Design review of the part built by this model. Coordinates are the model's own, in mm. A direction names the side the tool comes from. Coordinates: 2 decimals unless noted, no trailing zeros. Loops run counter-clockwise (first coordinate to the right, second up) from the corner with the lowest first, then second, coordinate; pieces in that order, holes last. Notation, with made-up numbers: (-1, 6) -> (50, 6) arc R37 ccw to (50, 43) -> close; hole circle Ø10 at (-35, -28.75). An arc over 180 degrees is marked (long way). One line per item, written item: value. Start each with the question number.
1. For probe 1 along Y at (x, z) = (0, 9.5); probe 2 along X at (y, z) = (-5.75, 33); probe 3 along Y at (x, z) = (3.25, 33.5), list the stretches that pass through material, from the lowest coordinate up.
2. Add section D-D on y = -5.5. Write out the cut boundary in (x, z), plus the area to 3 significant figures.
3. Machinability: for faces 1 (the cylindrical face through (0.07, 8.45, 18.54)), 2 (the flat face through (4.733, -4, 19)), 3 (the flat face through (-4.733, 4, 19)), 4 (the flat face through (-4.733, -4, 19)), 5 (the flat face through (4.733, 4, 19)), which of the approach directions +Z, -Z, +X, -X, +Y, -Y give a long, thin tool a straight path to every point of the face, cutting with its end or side? Answer none if there is none.
4. Draft analysis for pull direction X (two halves, no side actions). For faces 6 (the cylindrical face through (-5.458, -0.016, 19.063)), 7 (the cylindrical face through (-0.07, -8.45, 18.54)), 8 (the cylindrical face through (5.458, -0.016, 19.063)), 9 (the cylindrical face through (3.434, 1.081, 18.537)), state which applies: pulls with the +X half, pulls with the -X half, needs draft (parallel to the pull), parting line crosses it, or undercut.
5. Add section A-A on y = 0. Write out the cut boundary in (x, z), plus the area to 3 significant figures.
6. Insertion check: pin 1 (5 mm diameter, centred on y = 3, z = 11.5, fed in from +X); pin 2 (3 mm diameter, centred on y = -3, z = 21.5, fed in from -X); pin 3 (5 mm diameter, centred on y = 3, z = 13, fed in from -X); pin 4 (6 mm diameter, centred on x = 0, y = 0, fed in from +Z). Each pin has a flat end and moves straight along its axis. Give the tip position at first contact, or say it passes through.
7. Add section B-B on x = 0. Write out the cut boundary in (y, z).
8. Add section C-C on z = 26. Write out the cut boundary in (x, y) (3 decimals).
```python
from build123d import *

# Parameters (mm, degrees)
F0_R     = 3.6
F1_DEPTH = 37.6
F2_R     = 0.725
F3_DEPTH = 37.6


# Not quite as in the source:
# - a pattern or mirror of a feature is missing from the dataset's text; its kind, count and spacing are read off the source's solid


with BuildPart() as f1:
    # F0 (on Top) → F1 (new body)
    with BuildSketch(Plane.XY):
        with BuildLine():
            Line((4.7331279298, -7), (4.7331279298, 7))
            ThreePointArc((4.7331279298, 7), (0, 8.45), (-4.7331279298, 7))
            Line((-4.7331279298, 7), (-4.7331279298, -7))
            ThreePointArc((-4.7331279298, -7), (0, -8.45), (4.7331279298, -7))
        make_face()
        Circle(F0_R, mode=Mode.SUBTRACT)
    extrude(amount=F1_DEPTH)

    # F2 (on face) → F3 (join)
    with BuildSketch(Plane.XY.offset(37.6)):
        with Locations((4.7331279298, 0)):
            Circle(F2_R)
    f3 = extrude(amount=-F3_DEPTH)

    # F3_copies: F3 across plane
    add(f3.mirror(Plane(origin=(0, 0, 0), x_dir=(0, 0, -1), z_dir=(-1, 0, 0))))


solid = f1.part
```
Worked answers:
1. probe 1: y = -8.45 to -3.6, 3.6 to 8.45
1. probe 2: x = -4.73 to 4.73
1. probe 3: y = -7.8 to -1.55, 1.55 to 7.8
2. outline: (-4.73, 0) -> (4.73, 0) -> (4.73, 37.6) -> (-4.73, 37.6) -> close
2. area: 356 mm²
3. face 1: +Z, -Z, +Y
3. face 2: +Z, -Z, +X, -Y
3. face 3: +Z, -Z, -X, +Y
3. face 4: +Z, -Z, -X, -Y
3. face 5: +Z, -Z, +X, +Y
4. face 6: pulls with the -X half
4. face 7: parting line crosses it
4. face 8: pulls with the +X half
4. face 9: undercut
5. outline: (-5.46, 0) -> (-3.6, 0) -> (-3.6, 37.6) -> (-5.46, 37.6) -> close; (3.6, 0) -> (5.46, 0) -> (5.46, 37.6) -> (3.6, 37.6) -> close
5. area: 140 mm²
6. pin 1: stops at x = 5.26
6. pin 2: stops at x = -4.73
6. pin 3: stops at x = -5.26
6. pin 4: passes through
7. outline: (-8.45, 0) -> (-3.6, 0) -> (-3.6, 37.6) -> (-8.45, 37.6) -> close; (3.6, 0) -> (8.45, 0) -> (8.45, 37.6) -> (3.6, 37.6) -> close
8. outline: (-4.733, -7) arc R8.45 ccw to (4.733, -7) -> (4.733, -0.725) arc R0.725 ccw to (4.733, 0.725) -> (4.733, 7) arc R8.45 ccw to (-4.733, 7) -> (-4.733, 0.725) arc R0.725 ccw to (-4.733, -0.725) -> close; hole circle Ø7.2 at (0, 0)
